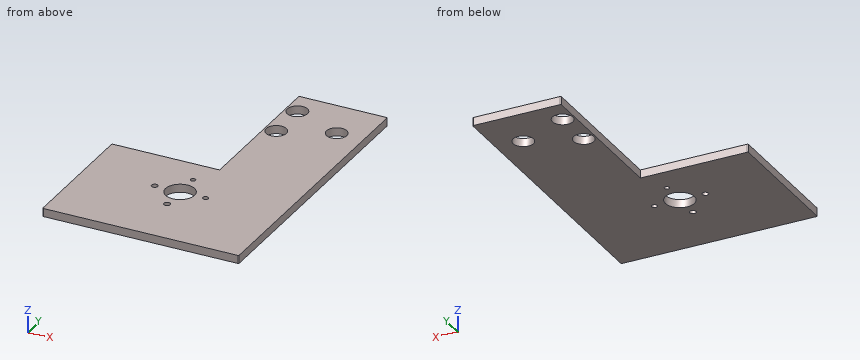
from build123d import *

# Parameters (mm, degrees)
SKETCH_1_R          = 10
SKETCH_1_R_2        = 14.237670301
EXTRUDE_1_DEPTH     = 8
SKETCH_2_R          = 2.388792686
SKETCH_2_R_2        = 2.719652574
SKETCH_2_R_3        = 3.086328998
SKETCH_2_R_4        = 2.978260763
CUT_EXTRUDE_1_DEPTH = 9


with BuildPart() as part:
    # 草图1 → 凸台-拉伸1 (new body)
    with BuildSketch(Plane.XY):
        with BuildLine():
            Line((4236.361201479, 3653.279497209), (4045.920724491, 3653.279497209))
            ThreePointArc((4045.920724491, 3653.279497209), (4045.21361771, 3653.572390428), (4044.920724491, 3654.279497209))
            Line((4044.920724491, 3654.279497209), (4044.920724491, 3785.62643227))
            ThreePointArc((4044.920724491, 3785.62643227), (4045.21361771, 3786.333539051), (4045.920724491, 3786.62643227))
            Line((4045.920724491, 3786.62643227), (4150.606085218, 3786.62643227))
            Line((4150.606085218, 3786.62643227), (4150.606085218, 3938.288234625))
            ThreePointArc((4150.606085218, 3938.288234625), (4150.898978436, 3938.995341406), (4151.606085218, 3939.288234625))
            Line((4151.606085218, 3939.288234625), (4236.361201479, 3939.288234625))
            ThreePointArc((4236.361201479, 3939.288234625), (4237.06830826, 3938.995341406), (4237.361201479, 3938.288234625))
            Line((4237.361201479, 3938.288234625), (4237.361201479, 3654.279497209))
            ThreePointArc((4237.361201479, 3654.279497209), (4237.06830826, 3653.572390428), (4236.361201479, 3653.279497209))
        make_face()
        with Locations((4210.911253899, 3893.629242063)):
            Circle(SKETCH_1_R, mode=Mode.SUBTRACT)
        with Locations((4161.960456262, 3913.970224185)):
            Circle(SKETCH_1_R, mode=Mode.SUBTRACT)
        with Locations((4161.960456262, 3873.288259941)):
            Circle(SKETCH_1_R, mode=Mode.SUBTRACT)
        with Locations((4138.223317867, 3734.818667022)):
            Circle(SKETCH_1_R_2, mode=Mode.SUBTRACT)
    extrude(amount=EXTRUDE_1_DEPTH)

    # 草图2 → 切除-拉伸1 (cut, through all)
    with BuildSketch(Plane.XY.offset(8)):
        with Locations((4138.223317867, 3759.818667022)):
            Circle(SKETCH_2_R)
        with Locations((4163.223317867, 3734.818667022)):
            Circle(SKETCH_2_R_2)
        with Locations((4138.223317867, 3709.818667022)):
            Circle(SKETCH_2_R_3)
        with Locations((4113.223317867, 3734.818667022)):
            Circle(SKETCH_2_R_4)
    extrude(amount=-CUT_EXTRUDE_1_DEPTH, mode=Mode.SUBTRACT)


solid = part.part
Verification items for the finished model (mm, model axes). Give positions to 0.01 mm unless a question says otherwise; leave off trailing zeros. Loops run counter-clockwise (first coordinate to the right, second up) from the corner with the lowest first, then second, coordinate; pieces in that order, holes last.
1) Thickness scan on line 1 along Y through (x, z) = (4113, 4.5); line 2 along X through (y, z) = (3914.5, 3.5); line 3 along X through (y, z) = (3789.5, 4.5). Record the ranges inside material, lowest first.
2) Sectioned sample at B-B, the plane x = 4071.5. Enter the section's corners in (y, z).
3) Depth check by flat-ended pin: pin 1 Ø2 at (x, y) = (4162, 3682) entering from -Z; pin 2 Ø4.5 at (x, y) = (4163.22, 3734.82) entering from +Z. Enter the tip coordinate at first touch or a pass-through.
4) Sectioned sample at A-A, the plane z = 6.5. Count the separate pieces of the cut face and the enclosed holes in it, then the cut area to 3 significant figures.
5) Sectioned sample at C-C, the plane y = 3815.5. Enter the section's corners in (x, z).
Answers:
1. line 1: y = 3653.28 to 3731.85, 3737.79 to 3786.63
1. line 2: x = 4150.61 to 4151.97, 4171.95 to 4237.36
1. line 3: x = 4150.61 to 4237.36
2. outline: (3653.28, 0) - (3786.63, 0) - (3786.63, 8) - (3653.28, 8) - close
3. pin 1: stops at z = 0
3. pin 2: passes through
4. separate pieces: 1
4. enclosed holes: 8
4. area: 37,200 mm2
5. outline: (4150.61, 0) - (4237.36, 0) - (4237.36, 8) - (4150.61, 8) - close
